For this review, take the finished solid that the model builds, in its own axes (mm). Coordinates: 2 decimals unless noted, no trailing zeros. Order: outer loops, then holes, each group sorted by start corner. A loop starts at its lowest first (then second) coordinate and runs counter-clockwise, first axis right, second up. Notation, with made-up numbers: (87.25, -24.75) -> (103.25, -24.75) arc R25 cw to (103.25, 10.25) -> close; hole circle Ø9 at (-16, 49). An arc over 180 degrees is marked (long way). Answer as a JSON object with one key per item and string values. Group by question number.
1) Draft analysis for pull direction X (two halves, no side actions). For faces 1 (the cylindrical face through (-46, 0, 8)), 2 (the flat face through (0, 29, 16)), 3 (the flat face through (51, 0, 8)), state which applies: +X half, -X half, draft (parallel to the pull), parting line (faces both ways), or undercut.
2) Add section D-D, the plane x = 40. Write out the cut boundary in (y, z).
3) Wall thickness on L1, parallel to X at y = -0.5, z = 15.5; L2, parallel to Y at x = 0, z = 27; L3, parallel to X at y = -1, z = 11.5: over which ranges is each line inside the solid? List them lowest first.
4) Add section A-A, the plane z = 12. Write out the cut boundary in (x, y), then the cut area to 3 significant figures.
5) For pin 1 (8 mm diameter, centred on x = 17, z = 11, fed in from -Y); pin 2 (12 mm diameter, centred on y = 13.5, z = 34, fed in from -X); pin 3 (4 mm diameter, centred on x = -33, y = 6, fed in from +Z); pin 4 (11 mm diameter, centred on x = -40, y = 0, fed in from +Z), all flat-tipped, find the tip position at first contact; note any pin that passes through.
6) Add section B-B, the plane x = 17. Write out the cut boundary in (y, z).
from build123d import *

# Parameters (mm, degrees)
F0_R     = 20
F1_DEPTH = 40
F0_R_2   = 6
F2_DEPTH = 16


with BuildPart() as f1:
    # F0 (on Top) → F1 (new body)
    with BuildSketch(Plane.XY):
        with BuildLine():
            ThreePointArc((10.26457, -26.050693), (23.14528, -15.757412), (28, 0))
            ThreePointArc((28, 0), (23.14528, 15.757412), (10.26457, 26.050693))
            ThreePointArc((10.26457, 26.050693), (0, 28), (-10.26457, 26.050693))
            ThreePointArc((-10.26457, 26.050693), (-28, 0), (-10.26457, -26.050693))
            ThreePointArc((-10.26457, -26.050693), (0, -28), (10.26457, -26.050693))
        make_face()
        Circle(F0_R, mode=Mode.SUBTRACT)
    extrude(amount=F1_DEPTH)

    # F0 (on Top) → F2 (join)
    with BuildSketch(Plane.XY):
        with BuildLine():
            ThreePointArc((10.26457, 26.050693), (23.14528, 15.757412), (28, 0))
            ThreePointArc((28, 0), (23.14528, -15.757412), (10.26457, -26.050693))
            Line((10.26457, -26.050693), (51, -10))
            Line((51, -10), (51, 10))
            Line((51, 10), (10.26457, 26.050693))
        make_face()
        with Locations((40, 0)):
            Circle(F0_R_2, mode=Mode.SUBTRACT)
        with BuildLine():
            ThreePointArc((-10.26457, 26.050693), (0, 28), (10.26457, 26.050693))
            Line((10.26457, 26.050693), (0, 30.095169))
            Line((0, 30.095169), (-10.26457, 26.050693))
        make_face()
        with BuildLine():
            Line((0, -30.095169), (10.26457, -26.050693))
            ThreePointArc((10.26457, -26.050693), (0, -28), (-10.26457, -26.050693))
            Line((-10.26457, -26.050693), (0, -30.095169))
        make_face()
        with BuildLine():
            ThreePointArc((-10.26457, -26.050693), (-28, 0), (-10.26457, 26.050693))
            Line((-10.26457, 26.050693), (-51, 10))
            Line((-51, 10), (-51, -10))
            Line((-51, -10), (-10.26457, -26.050693))
        make_face()
        with Locations((-40, 0)):
            Circle(F0_R_2, mode=Mode.SUBTRACT)
    extrude(amount=F2_DEPTH)


solid = f1.part
Output values:
{
 "1": {"face 1": "undercut", "face 2": "draft", "face 3": "+X half"},
 "2": {"outline": "(-14.33, 0) -> (-6, 0) -> (-6, 16) -> (-14.33, 16) -> close; (6, 0) -> (14.33, 0) -> (14.33, 16) -> (6, 16) -> close"},
 "3": {"L1": "x = -51 to -45.98, -34.02 to -19.99, 19.99 to 34.02, 45.98 to 51", "L2": "y = -28 to -20, 20 to 28", "L3": "x = -51 to -45.92, -34.08 to -19.97, 19.97 to 34.08, 45.92 to 51"},
 "4": {"outline": "(-51, -10) -> (0, -30.1) -> (51, -10) -> (51, 10) -> (0, 30.1) -> (-51, 10) -> close; hole circle Ø12 at (-40, 0); hole circle Ø40 at (0, 0); hole circle Ø12 at (40, 0)", "area": "2,610 mm²"},
 "5": {"pin 1": "stops at y = -24.97", "pin 2": "stops at x = -26.98", "pin 3": "stops at z = 16", "pin 4": "passes through"},
 "6": {"outline": "(-23.4, 0) -> (-10.54, 0) -> (-10.54, 40) -> (-22.25, 40) -> (-22.25, 16) -> (-23.4, 16) -> close; (10.54, 0) -> (23.4, 0) -> (23.4, 16) -> (22.25, 16) -> (22.25, 40) -> (10.54, 40) -> close"}
}
